Verification items for this drawing (mm, ordinates from the low corner). A direction names the side the tool comes from. Round coordinates to 2 decimals unless told otherwise and drop trailing zeros. Loops run counter-clockwise (first coordinate to the right, second up) from the corner with the lowest first, then second, coordinate; pieces in that order, holes last. Notation, with made-up numbers: (-34.5, 73.5) - (8.5, 73.5) arc R15 cw to (8.5, 79.5) - close; hole circle Ø6 at (59.5, 63). An arc over 180 degrees is marked (long way). Write item = value, one per line.
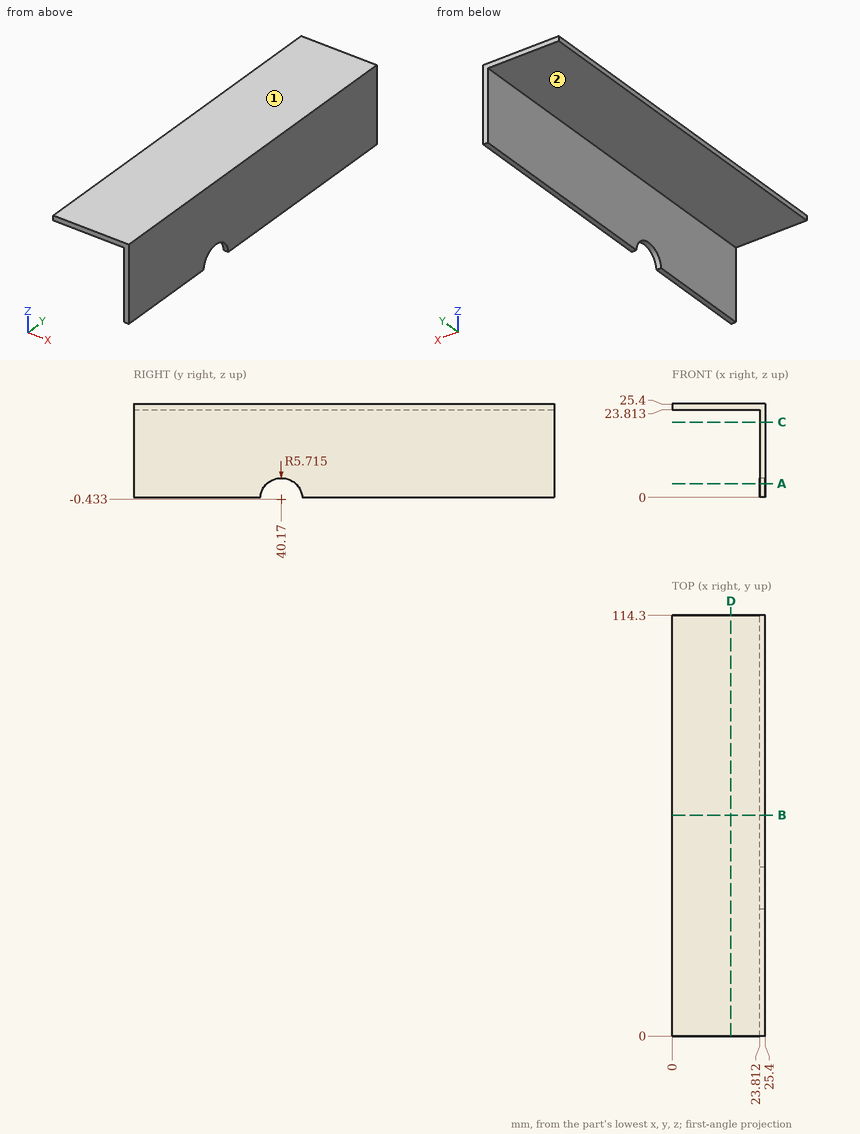
(1) Section check B-B (y = 60). Enter the section's corners in (x, z).
Answers follow:
outline = (0, 23.81) - (23.81, 23.81) - (23.81, 0) - (25.4, 0) - (25.4, 25.4) - (0, 25.4) - close
(2) Set-up check for the marked faces 1 and 2: record each of +Z, -Z, +X, -X, +Y, -Y from which the full face is reachable in a straight line by a thin tool's end or side.
Answers follow:
face_1 = +Z, +X, -X, +Y, -Y
face_2 = -Z, -X, +Y, -Y
(3) Section check A-A (z = 3.75). Enter the section's corners in (x, y), then the cut area to 3 significant figures.
Answers follow:
outline = (23.81, 0) - (25.4, 0) - (25.4, 36.28) - (23.81, 36.28) - close; (23.81, 44.06) - (25.4, 44.06) - (25.4, 114.3) - (23.81, 114.3) - close
area = 169 mm²
(4) Gauge pin test, flat ends, axial feed: pin 1 (3 mm diameter, centred on x = 6, y = 33.5, fed in from -Z); pin 2 (6 mm diameter, centred on y = 49.5, z = 9, fed in from -X). Record the tip position at first contact, or that the pin passes through.
Answers follow:
pin_1 = 23.81
pin_2 = 23.81
(5) Section check D-D (x = 16). Enter the section's corners in (y, z).
Answers follow:
outline = (0, 23.81) - (114.3, 23.81) - (114.3, 25.4) - (0, 25.4) - close
(6) Section check C-C (z = 20.5). Enter the section's corners in (x, y).
Answers follow:
outline = (23.81, 0) - (25.4, 0) - (25.4, 114.3) - (23.81, 114.3) - close
(7) Scan line: L1, parallel to X at y = 56, z = 16. Record every from-to range of solid material in increasing order. Write a range as [from, to].
Answers follow:
L1 = [23.81, 25.4]
